Here's how the part is built. I have some questions about the finished solid (model axes, mm). Face numbers are marked on the shaded views. Give positions to 0.01 mm unless a question says otherwise; leave off trailing zeros. Order: outer loops, then holes, each group sorted by start corner. A loop starts at its lowest first (then second) coordinate and runs counter-clockwise, first axis right, second up.
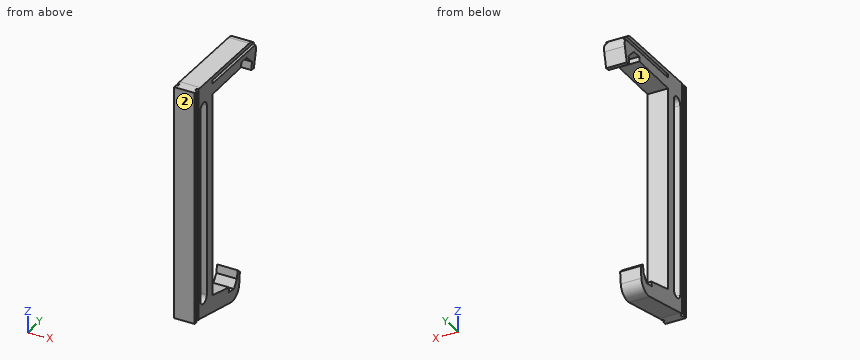
from build123d import *

# Parameters (mm, degrees)
BOSS_EXTRUDE1_DEPTH = 10
CUT_EXTRUDE4_REACH  = 126.4
CUT_EXTRUDE5_DEPTH  = 120.20766697


with BuildPart() as part:
    # Sketch1 → Boss-Extrude1 (new body)
    with BuildSketch(Plane(origin=(0, 0, 0), x_dir=(0, 0, -1), z_dir=(1, 0, 0))):
        with BuildLine():
            Line((0, 0), (100, 0))
            Line((100, 0), (103.946990438, 14.730368851))
            Line((103.946990438, 14.730368851), (106.217403847, 14.362642119))
            Line((106.217403847, 14.362642119), (106.952857311, 18.903468939))
            Line((106.952857311, 18.903468939), (103.341565092, 21.580990302))
            Line((103.341565092, 21.580990302), (99.393020031, 22.220515053))
            Line((99.393020031, 22.220515053), (101.210603817, 24.179837998))
            Line((101.210603817, 24.179837998), (107.020951621, 23.60910455))
            ThreePointArc((107.020951621, 23.60910455), (111.310577018, 21.133985308), (112.278030397, 16.276914661))
            Line((112.278030397, 16.276914661), (106, -10.68))
            Line((106, -10.68), (106, -15.68))
            Line((106, -15.68), (-9, -15.68))
            Line((-9, -15.68), (-9, -10.68))
            Line((-9, -10.68), (-8.111602248, 32.45071604))
            ThreePointArc((-8.111602248, 32.45071604), (-5.794866244, 37.064553263), (-0.751946881, 38.17077383))
            Line((-0.751946881, 38.17077383), (6.44531119, 36.494595175))
            Line((6.44531119, 36.494595175), (6.242876448, 34.365871735))
            Line((6.242876448, 34.365871735), (2.263353613, 34.770096924))
            Line((2.263353613, 34.770096924), (-2.28822563, 30.082429484))
            Line((-2.28822563, 30.082429484), (-2.28822563, 25.482429484))
            Line((-2.28822563, 25.482429484), (0, 25.25))
            Line((0, 25.25), (0, 0))
        make_face()
        with BuildLine():
            Line((2.84, -5), (97.16, -5))
            ThreePointArc((97.16, -5), (100, -7.84), (97.16, -10.68))
            Line((97.16, -10.68), (2.84, -10.68))
            ThreePointArc((2.84, -10.68), (0, -7.84), (2.84, -5))
        make_face(mode=Mode.SUBTRACT)
    extrude(amount=BOSS_EXTRUDE1_DEPTH)

    # Cut-Extrude4: up to this plane
    cut_extrude4_end = Plane(origin=(0, 0, 0), z_dir=(0, 1, 0))
    # Sketch2 → Cut-Extrude4 (cut, up to the surface)
    with BuildSketch(Plane(origin=(0, 38.268671352, -0.788250341), x_dir=(1, 0, 0), z_dir=(0, 0.9997879328481811, -0.020593429320073266)), mode=Mode.PRIVATE) as cut_extrude4_sk1:
        with BuildLine():
            Line((0, -5.291493544), (0, -6.964813597))
            ThreePointArc((0, -6.964813597), (1, -6.12815357), (0, -5.291493544))
        make_face()
    cut_extrude4_tool1 = split(extrude(cut_extrude4_sk1.sketch, amount=-CUT_EXTRUDE4_REACH, mode=Mode.PRIVATE), bisect_by=cut_extrude4_end, keep=Keep.BOTH, mode=Mode.PRIVATE)
    cut_extrude4 = cut_extrude4_tool1.solids().sort_by_distance((0.431182, 38.394871, 5.338604))[0]
    add(cut_extrude4, mode=Mode.SUBTRACT)

    # Mirror1: Cut-Extrude4 across plane
    add(cut_extrude4.mirror(Plane(origin=(5, 0, 0), x_dir=(0, 0, 1), z_dir=(1, 0, 0))), mode=Mode.SUBTRACT)

    # Sketch3 → Cut-Extrude5 (cut, symmetric)
    with BuildSketch(Plane.XY):
        with BuildLine():
            ThreePointArc((0, -13.866660027), (1, -13.03), (0, -12.193339973))
            Line((0, -12.193339973), (0, -13.866660027))
        make_face()
    cut_extrude5 = extrude(amount=CUT_EXTRUDE5_DEPTH, both=True, mode=Mode.SUBTRACT)

    # Mirror2: Cut-Extrude5 across plane
    add(cut_extrude5.mirror(Plane(origin=(5, 0, 0), x_dir=(0, 0, 1), z_dir=(1, 0, 0))), mode=Mode.SUBTRACT)


solid = part.part
Q1. I'm going to push flat-ended pins straight in: P1, Ø5, axis at x = 7.5, z = -52, coming from the +Y side; P2, Ø2.5, axis at x = 4, y = 27.5, coming from the -Z side; P3, Ø1.5, axis at x = 7, y = 30, coming from the -Z side. Where does each tip first touch, or does it pass through?
Filled sheet:
P1: stops at y = 0
P2: stops at z = 2.29
P3: stops at z = 1.64
Q2. I need wall thicknesses on L1, parallel to Y at x = 9.85, z = -27.5; L2, parallel to Y at x = 5.75, z = -91.5; L3, parallel to Y at x = 9.5, z = -36. Which ranges of each line are inside material? Lowest first, please.
Filled sheet:
L1: y = -15.68 to -13.88, -12.18 to -10.68, -5 to 0
L2: y = -15.68 to -10.68, -5 to 0
L3: y = -15.68 to -13.8, -12.26 to -10.68, -5 to 0
Q3. If we section it at A-A on z = -53.5: List the corners of the cut face in (x, y) for me.
Filled sheet:
outline: (0, -15.68) - (10, -15.68) - (10, -13.87) arc R0.85 cw (long way) to (10, -12.19) - (10, -10.68) - (0, -10.68) - (0, -12.19) arc R0.85 cw (long way) to (0, -13.87) - close; (0, -5) - (10, -5) - (10, 0) - (0, 0) - close
Q4. If we section it at C-C on y = -7.84: List the corners of the cut face in (x, z) for me.
Filled sheet:
outline: (0, -106.66) - (10, -106.66) - (10, -100) - (0, -100) - close; (0, 0) - (10, 0) - (10, 8.94) - (0, 8.94) - close
Q5. If we section it at B-B on x = 3: List the corners of the cut face in (y, z) for me, plus the area to 3 significant figures.
Filled sheet:
outline: (-15.68, -106) - (-10.68, -106) - (16.28, -112.28) arc R6 ccw to (23.61, -107.02) - (24.18, -101.21) - (22.22, -99.39) - (21.58, -103.34) - (18.9, -106.95) - (14.36, -106.22) - (14.73, -103.95) - (0, -100) - (0, 0) - (25.25, 0) - (25.48, 2.29) - (30.08, 2.29) - (34.77, -2.26) - (34.37, -6.24) - (36.49, -6.45) - (38.17, 0.75) arc R6 ccw to (32.45, 8.11) - (-10.68, 9) - (-15.68, 9) - close; hole (-10.68, -97.16) arc R2.84 ccw to (-5, -97.16) - (-5, -2.84) arc R2.84 ccw to (-10.68, -2.84) - close
area: 1,760 mm2
Q6. Thinking about a two-plate mould opening in Y: for the marked faces 1 and 2, which applies, released by +Y, released by -Y, zero draft, split by the parting line, or undercut?
Filled sheet:
face 1: undercut
face 2: released by -Y
